The drawing under review shows one solid part. Ordinate dimensions are in mm from its lowest x, y, z. Round coordinates to 2 decimals unless told otherwise and drop trailing zeros. Write each loop counter-clockwise with the first axis right and the second up, starting at its lowest first coordinate (ties: lowest second). Pieces come first, ordered by that corner, then holes. Notation, with made-up numbers: M 57,0.5 L 99,0.5 A21 ccw 99,8.5 Z; hole C 12.25,-31 d10. An arc over 180 degrees is marked long. One line per item, written item: value. Start each with the question number.
1) Take a section at C-C, the plane y = 13.25. Write out the cut boundary in (x, z), and give its area (3 significant figures).
2) For P1, Ø5, axis at y = 9, z = 19, coming from the +X side; P2, Ø5, axis at x = 8, z = 54, coming from the +Y side; P3, Ø1, axis at y = 14.5, z = 73.5, coming from the -X side, all flat-tipped, find the tip position at first contact; note any pin that passes through.
3) Wall thickness on probe 1 along X at (y, z) = (7.5, 49); probe 2 along Z at (x, y) = (12.5, 2.75); probe 3 along Y at (x, z) = (7.25, 20.5): over which ranges is each line inside the solid? List them lowest first.
4) Take a section at D-D, the plane z = 32. Write out the cut boundary in (x, y).
5) Take a section at A-A, the plane x = 7.5. Write out the cut boundary in (y, z), and give its area (3 significant figures).
6) Take a section at B-B, the plane y = 7.5. Write out the cut boundary in (x, z).
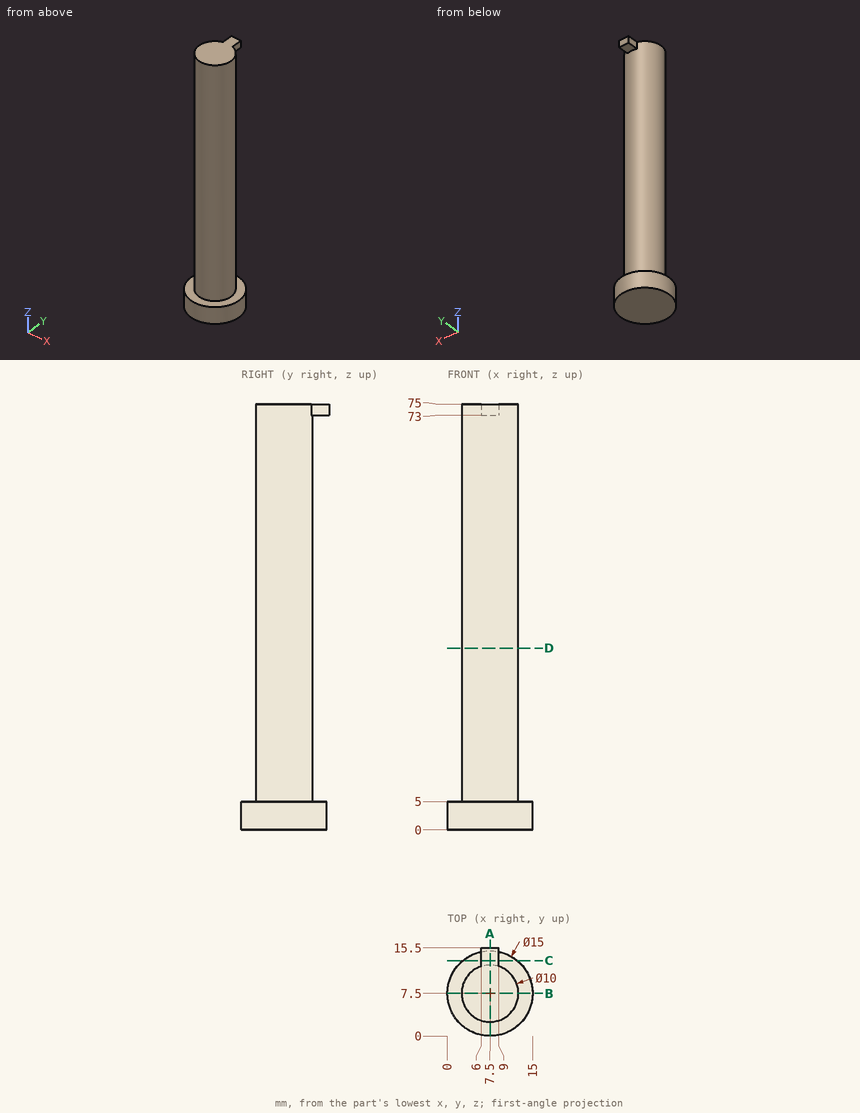
Checked values:
1. outline: M 2.68,0 L 12.32,0 L 12.32,5 L 2.68,5 Z; M 6,73 L 9,73 L 9,75 L 6,75 Z
1. area: 54.2 mm2
2. P1: stops at x = 12.5
2. P2: stops at y = 12.5
2. P3: stops at x = 6
3. probe 1: x = 2.5 to 12.5
3. probe 2: z = 0 to 5
3. probe 3: y = 2.51 to 12.49
4. outline: C 7.5,7.5 d10
5. outline: M 0,0 L 15,0 L 15,5 L 12.5,5 L 12.5,73 L 15.5,73 L 15.5,75 L 2.5,75 L 2.5,5 L 0,5 Z
5. area: 781 mm2
6. outline: M 0,0 L 15,0 L 15,5 L 12.5,5 L 12.5,75 L 2.5,75 L 2.5,5 L 0,5 Z
